For this review, take the finished solid that the model builds, in its own axes (mm). Give positions to 0.01 mm unless a question says otherwise; leave off trailing zeros. Order: outer loops, then holes, each group sorted by start corner. A loop starts at its lowest first (then second) coordinate and runs counter-clockwise, first axis right, second up.
Item 1: Consider section B-B (y = -0.85). Give the number of separate pieces and of enclosed holes in the cut face, plus the area to 3 significant figures.
Item 2: For P1, Ø2.5, axis at x = -6.095, z = -2.5, coming from the +Y side; P2, Ø0.8, axis at x = 63, y = -0.5, coming from the -Z side, all flat-tipped, find the tip position at first contact; note any pin that passes through.
Item 3: Consider section A-A (z = -17.6). Give the boundary of the cut face in (x, y) (3 decimals).
Item 4: For probe 1 along Z at (x, y) = (46.5, -0.85); probe 2 along Z at (x, y) = (56.5, -0.75); probe 3 along Z at (x, y) = (-10, -0.4), list the stretches that pass through material, from the lowest coordinate up.
Item 5: Consider section D-D (x = 24). Give the boundary of the cut face in (y, z).
Item 6: Consider section C-C (z = -9.98). Give the boundary of the cut face in (x, y), plus the area to 3 significant figures.
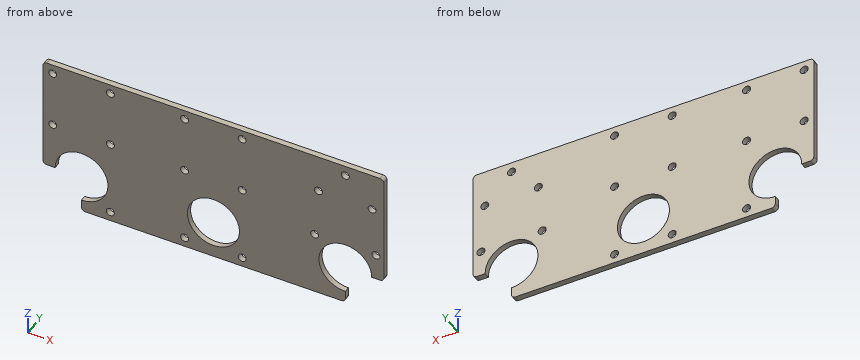
Autodesk Inventor part; units mm, degrees
ref_plane "YZ Plane" through (0, 0, 0) normal (1, 0, 0) x (0, 1, 0)
ref_plane "XZ Plane" through (0, 0, 0) normal (0, 1, 0) x (-1, 0, 0)
ref_plane "XY Plane" through (0, 0, 0) normal (0, 0, 1) x (1, 0, 0)
sketch "Sketch1" plane through (0, 0, 0) normal (0, 1, 0) x (-1, 0, 0)
  line L0 (-0.4496, -40.1) -> (-0.4496, 0)
  line L1 (-41.2289, 0) -> (-41.2289, -40.1)
  circle A0 centre (-20.8393, -30.1) radius 6.8
  circle A1 centre (-13.3143, -37.6) radius 1.05
  circle A2 centre (-28.3643, -37.6) radius 1.05
  circle A3 centre (-13.3143, -17.6) radius 1.05
  circle A4 centre (-28.3643, -17.6) radius 1.05
  circle A5 centre (-13.3143, -2.5) radius 1.05
  circle A6 centre (-28.3643, -2.5) radius 1.05
  circle A7 centre (6.095, -37.6) radius 1.05
  circle A8 centre (21.145, -17.6) radius 1.05
  circle A9 centre (6.095, -17.6) radius 1.05
  circle A10 centre (21.145, -2.5) radius 1.05
  circle A11 centre (6.095, -2.5) radius 1.05
  circle A12 centre (-47.2986, -23.2) radius 1.05
  circle A13 centre (-63.2986, -23.2) radius 1.05
  circle A14 centre (-48.2986, -9.98) radius 1.05
  circle A15 centre (-62.2986, -9.98) radius 1.05
  circle A16 centre (-55.2986, -2.68) radius 1.05
  arc A17 (23.69, -1) -> (22.69, 0) centre (22.69, -1) ccw
  arc A18 (-64.3686, 0) -> (-65.3686, -1) centre (-64.3686, -1) ccw
  line L2 (-65.3686, -29.1) -> (-65.3686, -1)
  arc A19 (-65.3686, -29.1) -> (-64.3686, -30.1) centre (-64.3686, -29.1) ccw
  line L3 (-64.3686, -30.1) -> (-62.1986, -30.1)
  arc A20 (-55.2986, -39.1) -> (-54.2986, -40.1) centre (-54.2986, -39.1) ccw
  line L4 (-55.2986, -37) -> (-55.2986, -39.1)
  arc A21 (22.69, -30.1) -> (23.69, -29.1) centre (22.69, -29.1) ccw
  line L5 (20.52, -30.1) -> (22.69, -30.1)
  arc A22 (12.62, -40.1) -> (13.62, -39.1) centre (12.62, -39.1) ccw
  line L6 (13.62, -39.1) -> (13.62, -37)
  arc A23 (20.52, -30.1) -> (13.62, -37) centre (13.62, -30.1) ccw
  arc A24 (-55.2986, -37) -> (-62.1986, -30.1) centre (-55.2986, -30.1) ccw
  line L7 (23.69, -1) -> (23.69, -29.1)
  line L8 (-64.3686, 0) -> (22.69, 0)
  line L9 (12.62, -40.1) -> (-54.2986, -40.1)
  line L10 (-41.6786, -40.1) -> (-41.6786, 0)
  line L11 (-40.7793, 0) -> (-40.7793, -40.1)
  line L12 (-0.8993, -40.1) -> (-0.8993, 0)
  line L13 (0, 0) -> (0, -40.1)
  point P0 (0, 0)
extrude "Extrusion1" add sketch "Sketch1" against normal blind 1.5
properties part number "axis_5_top_frame" material "Aluminum 6061-AHC"
Resolved:
1. separate pieces: 1
1. enclosed holes: 17
1. area: 2,940 mm2
2. P1: stops at y = 0
2. P2: stops at z = -30.1
3. outline: (-23.69, -1.5) - (-22.195, -1.5) - (-22.195, 0) - (-23.69, 0) - close; (-20.095, -1.5) - (-7.145, -1.5) - (-7.145, 0) - (-20.095, 0) - close; (-5.045, -1.5) - (12.264, -1.5) - (12.264, 0) - (-5.045, 0) - close; (14.364, -1.5) - (27.314, -1.5) - (27.314, 0) - (14.364, 0) - close; (29.414, -1.5) - (65.369, -1.5) - (65.369, 0) - (29.414, 0) - close
4. probe 1: z = -40.1 to -23.88, -22.52 to 0
4. probe 2: z = -23.31 to 0
4. probe 3: z = -40.1 to -35.97, -24.23 to 0
5. outline: (-1.5, -40.1) - (0, -40.1) - (0, -36.12) - (-1.5, -36.12) - close; (-1.5, -24.08) - (0, -24.08) - (0, 0) - (-1.5, 0) - close
6. outline: (-23.69, -1.5) - (47.25, -1.5) - (47.25, 0) - (-23.69, 0) - close; (49.35, -1.5) - (61.25, -1.5) - (61.25, 0) - (49.35, 0) - close; (63.35, -1.5) - (65.37, -1.5) - (65.37, 0) - (63.35, 0) - close
6. area: 127 mm2
